Print and shaded views of the part. All mm, measured from the part's lowest x, y and z. A direction names the side the tool comes from. Give positions to 0.01 mm unless a question says otherwise; leave off trailing zeros. Loops run counter-clockwise (first coordinate to the right, second up) from the corner with the lowest first, then second, coordinate; pieces in that order, holes last. Notation, with made-up numbers: M -18.75,-14.75 L 0.25,-14.75 A9 ccw 0.25,-5.75 Z; hole C 56.25,32.5 d8. An arc over 180 degrees is marked long. Answer in a Markdown table with one row per item.
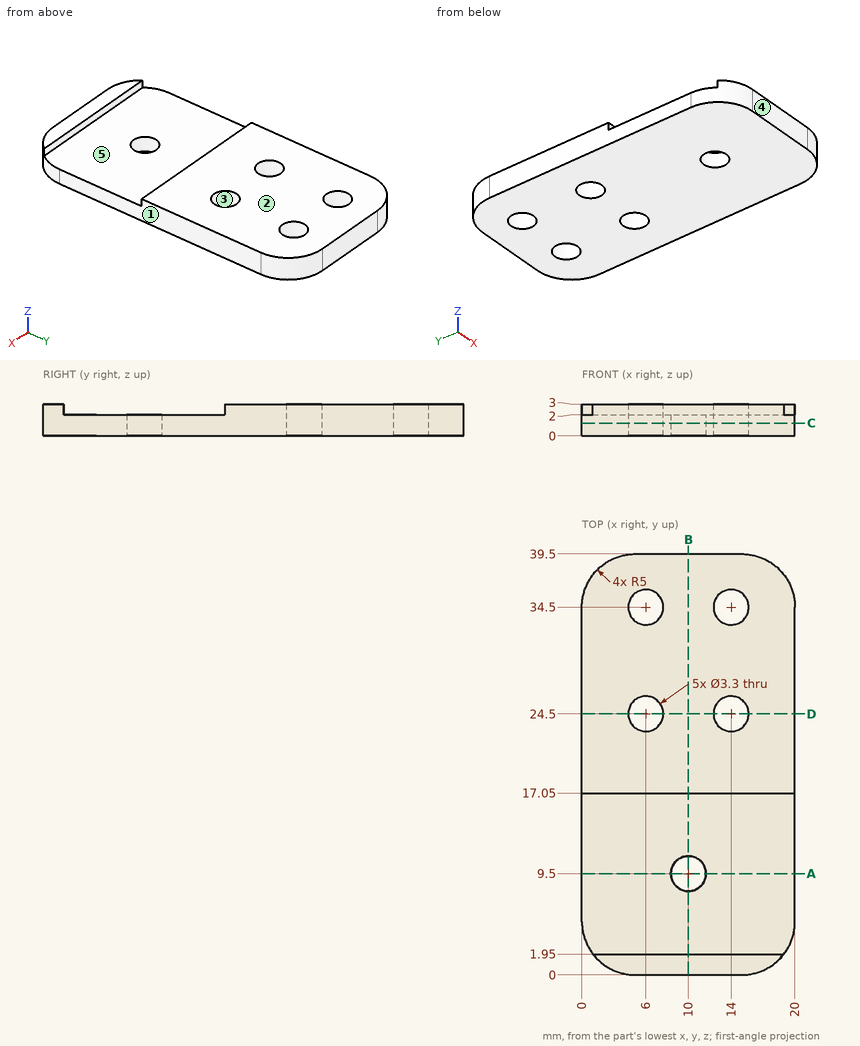
(1) Flat gauge pins, fed straight in: P1, Ø2.5, axis at x = 10, y = 9.5, coming from the +Z side; P2, Ø10, axis at x = 16.5, y = 12, coming from the +Z side. Where does each tip first touch, or does it go through?
Established:
| item | result |
|---|---|
| P1 | passes through |
| P2 | stops at z = 2 |
(2) Saw through at C-C, the plane z = 1.2. Give the cut face in (x, y), and give its area (3 significant figures).
Established:
| item | result |
|---|---|
| outline | M 0,5 A5 ccw 5,0 L 15,0 A5 ccw 20,5 L 20,34.5 A5 ccw 15,39.5 L 5,39.5 A5 ccw 0,34.5 Z; hole C 6,24.5 d3.3; hole C 6,34.5 d3.3; hole C 10,9.5 d3.3; hole C 14,24.5 d3.3; hole C 14,34.5 d3.3 |
| area | 726 mm2 |
(3) Saw through at B-B, the plane x = 10. Give the cut face in (y, z), and give its area (3 significant figures).
Established:
| item | result |
|---|---|
| outline | M 0,0 L 7.85,0 L 7.85,2 L 1.95,2 L 1.95,3 L 0,3 Z; M 11.15,0 L 39.5,0 L 39.5,3 L 17.05,3 L 17.05,2 L 11.15,2 Z |
| area | 96.8 mm2 |
(4) Saw through at A-A, the plane y = 9.5. Give the cut face in (x, z).
Established:
| item | result |
|---|---|
| outline | M 0,0 L 8.35,0 L 8.35,2 L 0,2 Z; M 11.65,0 L 20,0 L 20,2 L 11.65,2 Z |
(5) Saw through at D-D, the plane y = 24.5. Give the cut face in (x, z), and give its area (3 significant figures).
Established:
| item | result |
|---|---|
| outline | M 0,0 L 4.35,0 L 4.35,3 L 0,3 Z; M 7.65,0 L 12.35,0 L 12.35,3 L 7.65,3 Z; M 15.65,0 L 20,0 L 20,3 L 15.65,3 Z |
| area | 40.2 mm2 |
(6) Mould opens along X. For the marked faces 1, 2 and 3 say: pulls with the +X half, pulls with the -X half, needs draft (parallel to the pull), parting line crosses it, or undercut.
Established:
| item | result |
|---|---|
| face 1 | pulls with the +X half |
| face 2 | needs draft |
| face 3 | undercut |
(7) Which spindle directions (+Z, -Z, +X, -X, +Y, -Y) get a long thin tool onto all of the face, cutting with end or side? Do the marked faces 4 and 5. Say none if no direction does.
Established:
| item | result |
|---|---|
| face 4 | +Z, -Z, +X, -X, -Y |
| face 5 | +Z, +X, -X |
(8) Wall check: L1, parallel to Y at x = 6, z = 2.3; L2, parallel to Y at x = 6, z = 1.7; L3, parallel to Y at x = 14.75, z = 2.85. Give the ranges that are in metal, low to high.
Established:
| item | result |
|---|---|
| L1 | y = 0 to 1.95, 17.05 to 22.85, 26.15 to 32.85, 36.15 to 39.5 |
| L2 | y = 0 to 22.85, 26.15 to 32.85, 36.15 to 39.5 |
| L3 | y = 0 to 1.95, 17.05 to 23.03, 25.97 to 33.03, 35.97 to 39.5 |
